```python
from build123d import *

# Parameters (mm, degrees)
F1_R     = 25.4
F1_R_2   = 22.225
F2_DEPTH = 54.61
F3_R     = 3.81
F3_R_2   = 25.4
F4_DEPTH = 3.175
F5_R     = 6.35


with BuildPart() as f2:
    # F1 (on offset) → F2 (new body, symmetric)
    with BuildSketch(Plane.XZ.offset(9.525)):
        Circle(F1_R)
        Circle(F1_R_2, mode=Mode.SUBTRACT)
    extrude(amount=F2_DEPTH, both=True)

    # F3 (on Front) → F4 (join, symmetric)
    with BuildSketch(Plane.XZ):
        with BuildLine():
            ThreePointArc((42.8826136347, -11.6997413585), (44.0564108619, -5.902131985), (44.45, 0))
            ThreePointArc((44.45, 0), (44.0564108619, 5.902131985), (42.8826136347, 11.6997413585))
            ThreePointArc((42.8826136347, 11.6997413585), (22.0016274966, 22.0016274966), (11.6997413585, 42.8826136347))
            ThreePointArc((11.6997413585, 42.8826136347), (0, 44.45), (-11.6997413585, 42.8826136347))
            ThreePointArc((-11.6997413585, 42.8826136347), (-22.0016274966, 22.0016274966), (-42.8826136347, 11.6997413585))
            ThreePointArc((-42.8826136347, 11.6997413585), (-44.45, 0), (-42.8826136347, -11.6997413585))
            ThreePointArc((-42.8826136347, -11.6997413585), (-22.0016274966, -22.0016274966), (-11.6997413585, -42.8826136347))
            ThreePointArc((-11.6997413585, -42.8826136347), (0, -44.45), (11.6997413585, -42.8826136347))
            ThreePointArc((11.6997413585, -42.8826136347), (22.0016274966, -22.0016274966), (42.8826136347, -11.6997413585))
        make_face()
        with Locations((0, -34.925)):
            Circle(F3_R, mode=Mode.SUBTRACT)
        with Locations((-34.925, 0)):
            Circle(F3_R, mode=Mode.SUBTRACT)
        Circle(F3_R_2, mode=Mode.SUBTRACT)
        with Locations((34.925, 0)):
            Circle(F3_R, mode=Mode.SUBTRACT)
        with Locations((0, 34.925)):
            Circle(F3_R, mode=Mode.SUBTRACT)
    extrude(amount=F4_DEPTH, both=True)

    # F5
    f5_edges = [f2.edges().sort_by_distance(p)[0] for p in [
        (11.699741, 0, 42.882614),
        (-42.882614, 0, 11.699741),
        (-11.699741, 0, -42.882614),
        (42.882614, 0, -11.699741),
        (42.882614, 0, 11.699741),
        (-11.699741, 0, 42.882614),
        (-42.882614, 0, -11.699741),
        (11.699741, 0, -42.882614),
    ]]
    fillet(f5_edges, radius=F5_R)


solid = f2.part
```
Geometry check sheet. Reference: the model listing, model coordinates, mm. A direction names the side the tool comes from. Round coordinates to 2 decimals unless told otherwise and drop trailing zeros. Write each loop counter-clockwise with the first axis right and the second up, starting at its lowest first coordinate (ties: lowest second). Pieces come first, ordered by that corner, then holes. Notation, with made-up numbers: (39.25, 0) -> (71.25, 0) arc R9 cw to (71.25, 4) -> close; hole circle Ø2 at (85.5, -35). An arc over 180 degrees is marked (long way). Put each result on its own line as item: value.
1) Depth check by flat-ended pin: P1, Ø5, axis at y = -6.5, z = -13, coming from the +X side; P2, Ø10, axis at x = 34.925, z = 0, coming from the -Y side (3 decimals); P3, Ø1, axis at x = 22.5, y = -1, coming from the +Z side. Enter the tip coordinate at first touch or a pass-through.
Recorded:
P1: stops at x = 23.13
P2: stops at y = -3.175
P3: stops at z = 22
2) Cross-section at C-C, the plane x = 14.5. Enter the section's corners in (y, z) (1 decimal).
Recorded:
outline: (-64.1, -20.9) -> (-3.2, -20.9) -> (-3.2, -32.9) -> (3.2, -32.9) -> (3.2, -20.9) -> (45.1, -20.9) -> (45.1, -16.8) -> (-64.1, -16.8) -> close; (-64.1, 16.8) -> (45.1, 16.8) -> (45.1, 20.9) -> (3.2, 20.9) -> (3.2, 32.9) -> (-3.2, 32.9) -> (-3.2, 20.9) -> (-64.1, 20.9) -> close
3) Cross-section at A-A, the plane x = 0. Enter the section's corners in (y, z) (3 decimals).
Recorded:
outline: (-64.135, -25.4) -> (-3.175, -25.4) -> (-3.175, -31.115) -> (3.175, -31.115) -> (3.175, -25.4) -> (45.085, -25.4) -> (45.085, -22.225) -> (-64.135, -22.225) -> close; (-64.135, 22.225) -> (45.085, 22.225) -> (45.085, 25.4) -> (3.175, 25.4) -> (3.175, 31.115) -> (-3.175, 31.115) -> (-3.175, 25.4) -> (-64.135, 25.4) -> close; (-3.175, -44.45) -> (3.175, -44.45) -> (3.175, -38.735) -> (-3.175, -38.735) -> close; (-3.175, 38.735) -> (3.175, 38.735) -> (3.175, 44.45) -> (-3.175, 44.45) -> close
4) Cross-section at D-D, the plane y = 29. Enter the section's corners in (x, z) (3 decimals).
Recorded:
outline: circle Ø50.8 at (0, 0); hole circle Ø44.45 at (0, 0)
5) Cross-section at B-B, the plane z = 0. Enter the section's corners in (x, y) (3 decimals).
Recorded:
outline: (-44.45, -3.175) -> (-38.735, -3.175) -> (-38.735, 3.175) -> (-44.45, 3.175) -> close; (-31.115, -3.175) -> (-25.4, -3.175) -> (-25.4, -64.135) -> (-22.225, -64.135) -> (-22.225, 45.085) -> (-25.4, 45.085) -> (-25.4, 3.175) -> (-31.115, 3.175) -> close; (22.225, -64.135) -> (25.4, -64.135) -> (25.4, -3.175) -> (31.115, -3.175) -> (31.115, 3.175) -> (25.4, 3.175) -> (25.4, 45.085) -> (22.225, 45.085) -> close; (38.735, -3.175) -> (44.45, -3.175) -> (44.45, 3.175) -> (38.735, 3.175) -> close
6) Thickness scan on probe 1 along Y at (x, z) = (31, 7) (3 decimals); probe 2 along X at (y, z) = (-29, 16); probe 3 along Z at (x, y) = (-11.5, -43.5). Record the ranges inside material, lowest first. Write a range as from..to.
Recorded:
probe 1: y = -3.175..3.175
probe 2: x = -19.73..-15.43, 15.43..19.73
probe 3: z = -22.65..-19.02, 19.02..22.65
7) Access from +Z, -Z, +X, -X, +Y, -Y to the whole of each face (thin tool, end or side, straight path). Record for faces 1 (the face through (-17, 3.175, -20)), 2 (the face through (-0.1, -0.04, -44.45)).
Recorded:
face 1: +Y
face 2: -Z, +Y, -Y
8) Release check for a two-part mould opening along Z. For faces 3 (the face through (-5.506, -34.082, -24.796)), 4 (the face through (-22.199, -0.044, -21.806)), 5 (the face through (38.444, 0.044, -1.459)), 6 (the face through (-17, -3.175, -20)) record: pulls with the +Z half, pulls with the -Z half, needs draft (parallel to the pull), parting line crosses it, or undercut.
Recorded:
face 3: parting line crosses it
face 4: pulls with the -Z half
face 5: undercut
face 6: needs draft
